For this review, use the dimensioned drawing (mm, ordinates from the lowest corner) and the shaded views. A direction names the side the tool comes from. Give positions to 0.01 mm unless a question says otherwise; leave off trailing zeros. Write each loop counter-clockwise with the first axis right and the second up, starting at its lowest first coordinate (ties: lowest second). Pieces come first, ordered by that corner, then holes. Notation, with made-up numbers: M 69,-16 L 98,-16 A28 cw 98,15 Z; hole C 20,5 d6. An arc over 180 degrees is marked long. One line per item, written item: value. Start each with the question number.
Item 1: Consider section C-C, the plane x = 602. Write out the cut boundary in (y, z).
Item 2: Consider section B-B, the plane z = 22.5. Write out the cut boundary in (x, y), and give its area (3 significant figures).
Item 3: Clearance check with flat-ended pins moving along their axes: pin 1 Ø1 at (y, z) = (263, 220) entering from -X; pin 2 Ø3 at (x, z) = (720, 159.5) entering from +Y. State where each tip first meets the part, or that it passes through.
Item 4: To check wall thickness, follow probe 1 along X at (y, z) = (918, 159); probe 2 along Y at (x, z) = (503.5, 151.5). State the ranges of each line that lie inside material, in increasing order.
Item 5: Consider section A-A, the plane y = 737.5. Write out the cut boundary in (x, z), and give its area (3 significant figures).
Item 6: Tool access review of the marked faces 1 and 2: name each direction out of +Z, -Z, +X, -X, +Y, -Y from which nothing blocks a thin tool from reaching the whole face with its end or side.
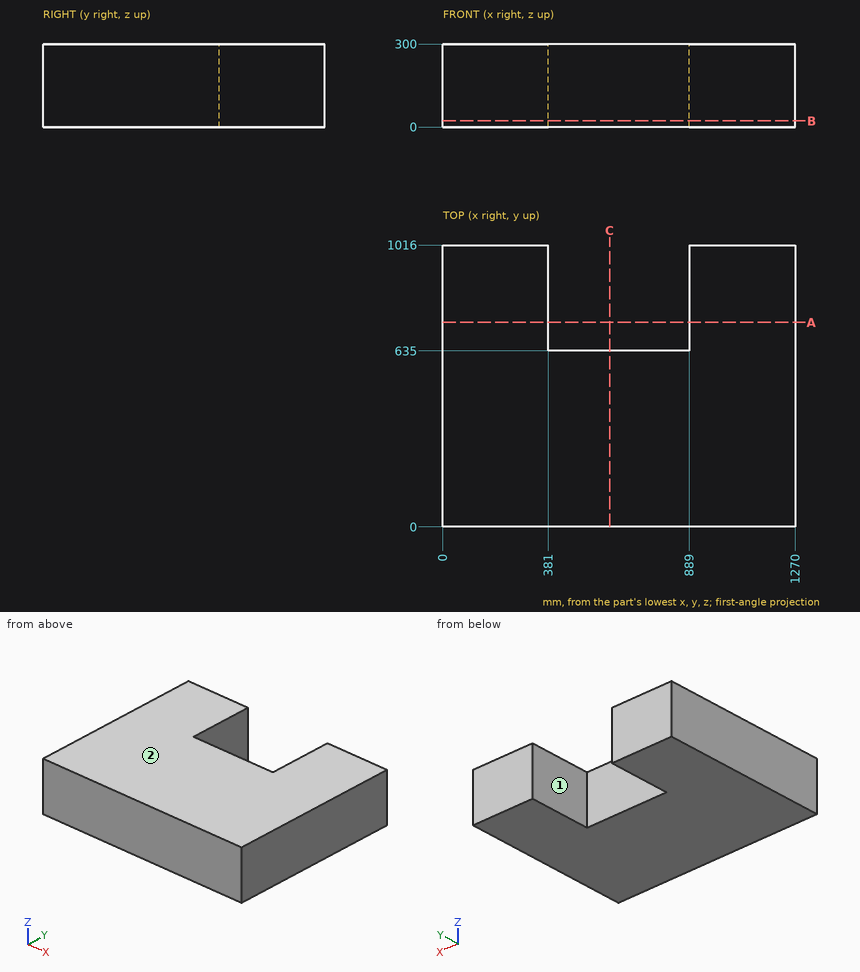
Model answer:
1. outline: M 0,0 L 635,0 L 635,300 L 0,300 Z
2. outline: M 0,0 L 1270,0 L 1270,1016 L 889,1016 L 889,635 L 381,635 L 381,1016 L 0,1016 Z
2. area: 1,100,000 mm2
3. pin 1: stops at x = 0
3. pin 2: stops at y = 635
4. probe 1: x = 0 to 381, 889 to 1270
4. probe 2: y = 0 to 635
5. outline: M 0,0 L 381,0 L 381,300 L 0,300 Z; M 889,0 L 1270,0 L 1270,300 L 889,300 Z
5. area: 229,000 mm2
6. face 1: +Z, -Z, +Y
6. face 2: +Z, +X, -X, +Y, -Y
